from build123d import *

# Parameters (mm, degrees)
F1_DEPTH = 46
F3_DEPTH = 16
F5_DEPTH = 46.001


# Not quite as in the source:
# - a feature names something its author has since deleted; it is built from what else it names


with BuildPart() as f1:
    # F0 (on Front) → F1 (new body)
    with BuildSketch(Plane.XZ):
        with BuildLine():
            ThreePointArc((0.1762595361, 0), (16.1762595361, -16), (32.1762595361, 0))
            Line((32.1762595361, 0), (0.1762595361, 0))
        make_face()
        with BuildLine():
            Line((0.1762595361, 0), (32.1762595361, 0))
            ThreePointArc((32.1762595361, 0), (16.1762595361, 16), (0.1762595361, 0))
        make_face()
        with BuildLine():
            ThreePointArc((0.1762595361, 0), (16.1762595361, 16), (32.1762595361, 0))
            Line((32.1762595361, 0), (32.3525190723, 0))
            Line((32.3525190723, 0), (32.3525190723, 14))
            Line((32.3525190723, 14), (32.3525190723, 30))
            Line((32.3525190723, 30), (0, 30))
            Line((0, 30), (0, 0))
            Line((0, 0), (0.1762595361, 0))
        make_face()
        Polygon((32.3525190723, 30), (32.3525190723, 14), (150.0428766012, 14), (150.0428766012, 30), (104.9743145704, 30), (67.9628998041, 30), (45.0152419508, 30), align=None)
    extrude(amount=F1_DEPTH)

    # F2 (on face) → F3 (cut)
    with BuildSketch(Plane.XY.offset(30)):
        Polygon((90.0428766012, 0), (150.0428766012, -8), (150.0428766012, 0), align=None)
        Polygon((90.0428766012, -46), (150.0428766012, -46), (150.0428766012, -38), align=None)
    extrude(amount=-F3_DEPTH, mode=Mode.SUBTRACT)

    # F4 (on face) → F5 (cut, through all)
    with BuildSketch(Plane.XY.offset(30)):
        with BuildLine():
            Line((86.5, -15), (68, -15))
            Line((68, -15), (49.5, -15))
            ThreePointArc((49.5, -15), (41.5, -23), (49.5, -31))
            Line((49.5, -31), (68, -31))
            Line((68, -31), (86.5, -31))
            ThreePointArc((86.5, -31), (94.5, -23), (86.5, -15))
        make_face()
    extrude(amount=-F5_DEPTH, mode=Mode.SUBTRACT)


solid = f1.part
Input: part model. Units: mm. Frame: model coordinates. A direction names the side the tool comes from. Give positions to 0.01 mm unless a question says otherwise; leave off trailing zeros. Order: outer loops, then holes, each group sorted by start corner. A loop starts at its lowest first (then second) coordinate and runs counter-clockwise, first axis right, second up. Notation, with made-up numbers: (71, 40.25) - (120, 40.25) arc R13 ccw to (120, 47.25) - close; hole circle Ø5 at (-34.5, -17). An arc over 180 degrees is marked (long way). Answer as a JSON object with one key per item and string values. Group by question number.
Q1. Cut plane D-D, the plane y = -36.5. Output: boundary loops of the cut face in (x, z).
Q2. Cut plane B-B, the plane x = 59. Output: boundary loops of the cut face in (y, z).
Q3. Line query: probe 1 along Z at (x, y) = (85, -36.5); probe 2 along X at (y, z) = (-16, 6.5); probe 3 along X at (y, z) = (-18.5, 19). Output: solid intervals per line, ascending.
Q4. Set-up query: faces 4 (the face through (94.498, -23.176, 22.112)), 5 (the face through (34, 0, 18)), 6 (the face through (32.353, -23, 7)). Return all of +Z, -Z, +X, -X, +Y, -Y with unobstructed straight access to the full face (end or side cutting, diameter ignored); none if empty.
Q5. Mould query, pull axis X, two halves, no side actions, for faces 1 (the face through (150.043, -23, 22)), 2 (the face through (68, -15, 22)), 3 (the face through (90, -33, 14)). Classes: pulls with the +X half, pulls with the -X half, needs draft (parallel to the pull), parting line crosses it, or undercut.
Q6. Cut plane C-C, the plane z = 16. Output: boundary loops of the cut face in (x, y), then the cut area to 3 significant figures.
Q7. First-contact query: pin 1 Ø1 at (y, z) = (-39.5, -7.5) entering from +X; pin 2 Ø3 at (y, z) = (-32, -2) entering from +X. Flat tips, straight axial feed; report the tip coordinate or a pass-through.
Q8. Cut plane A-A, the plane y = -23. Output: boundary loops of the cut face in (x, z), then the cut area to 3 significant figures.
Results:
{
 "1": {"outline": "(0, 0) - (0.18, 0) arc R16 ccw to (32.18, 0) - (32.35, 0) - (32.35, 14) - (150.04, 14) - (150.04, 30) - (0, 30) - close"},
 "2": {"outline": "(-46, 14) - (-31, 14) - (-31, 30) - (-46, 30) - close; (-15, 14) - (0, 14) - (0, 30) - (-15, 30) - close"},
 "3": {"probe 1": "14 to 30", "probe 2": "0 to 32.35", "probe 3": "0 to 42.89, 93.11 to 150.04"},
 "4": {"face 4": "+Z, -Z", "face 5": "+Z, -Z, +X, -X, +Y", "face 6": "-Z, +X, +Y, -Y"},
 "5": {"face 1": "pulls with the +X half", "face 2": "undercut", "face 3": "needs draft"},
 "6": {"outline": "(0, -46) - (90.04, -46) - (150.04, -38) - (150.04, -8) - (90.04, 0) - (0, 0) - close; hole (49.5, -31) - (86.5, -31) arc R8 ccw to (86.5, -15) - (49.5, -15) arc R8 ccw to start", "area": "5,630 mm^2"},
 "7": {"pin 1": "x = 30.56", "pin 2": "x = 32.17"},
 "8": {"outline": "(0, 0) - (0.18, 0) arc R16 ccw to (32.18, 0) - (32.35, 0) - (32.35, 14) - (41.5, 14) - (41.5, 30) - (0, 30) - close; (94.5, 14) - (150.04, 14) - (150.04, 30) - (94.5, 30) - close", "area": "2,410 mm^2"}
}
